Work out the finished part from the listing and answer in its coordinate system (mm). A direction names the side the tool comes from. Coordinates: 2 decimals unless noted, no trailing zeros. Write each loop counter-clockwise with the first axis right and the second up, starting at its lowest first coordinate (ties: lowest second). Pieces come first, ordered by that corner, then holes. Notation, with made-up numbers: (86, 81.25) - (121, 81.25) arc R17 ccw to (121, 102.25) - close; hole circle Ø1 at (-12, -20). An arc over 180 degrees is marked (long way). Use a Markdown table: item, result. Add a question column.
(1) For a pull along Z with two mould halves and no side action, classify faces 4 (the face through (37.236, 8, -89)), 5 (the face through (182.496, 124.457, -88.621)), 6 (the face through (187.325, 89, -83)) as released by +Z, released by -Z, zero draft, split by the parting line, or undercut.
(2) The part is cut by section B-B, the plane y = 84. Give the vertices of the cut face in (x, z) (3 decimals), then the cut area to 3 significant figures.
(3) The part is cut by section A-A, the plane x = 79. Give the vertices of the cut face in (y, z).
(4) A tool of negligible diameter and unlimited length cuts with its end or side. For faces 1 (the face through (185, 52.701, -89)), 2 (the face through (109, 8, -117.196)), 3 (the face through (83, 10.16, -66)), from which of +Z, -Z, +X, -X, +Y, -Y can it reach the whole face along a straight path? Write none if from no direction.
(5) Given pin 1 Ø17.5 at (y, z) = (99.5, -92.5) entering from +X (3 decimals); pin 2 Ø1.9 at (y, z) = (111.76, -88.9) entering from +X; pin 3 Ø12 at (y, z) = (65, -71) entering from -X; pin 4 Ø10 at (x, z) = (150, -111.5) entering from +Y, each flat-ended and moving along its own axis, determine where each tip first touches the part or whether it passes through.
(6) The part is cut by section C-C, the plane z = -139. Give the vertices of the cut face in (x, y), then the cut area to 3 significant figures.
(7) The part is cut by section D-D, the plane x = 23. Give the vertices of the cut face in (y, z).
(8) Find the intervals of material crossed by line 1 (Y direction, x = 185.25, z = -88.9); line 2 (Z direction, x = 39, y = 10); line 3 (Z direction, x = 181.5, y = 111.76), in increasing order. Write a range as from..to.
Autodesk Inventor part; units mm, degrees
ref_plane "Work Plane1" through (177.8, 10.16, -88.9) normal (0, 0, 1) x (1, 0, 0)
ref_plane "YZ Plane" through (0, 0, 0) normal (1, 0, 0) x (0, 1, 0)
ref_plane "XZ Plane" through (0, 0, 0) normal (0, 1, 0) x (-1, 0, 0)
sketch "Sketch1" plane through (0, 0, 0) normal (0, 1, 0) x (-1, 0, 0)
  line L0 (0, 0) -> (-203.2, 0)
  line L1 (-203.2, 0) -> (-203.2, -177.8)
  line L2 (-203.2, -177.8) -> (0, -177.8)
  line L3 (0, -177.8) -> (0, 0)
  dimension "d0" = 203.2
  dimension "d1" = 177.8
extrude "Extrusion1" add sketch "Sketch1" along normal blind 10.16
sketch "Sketch2" plane through (0, 10.16, 0) normal (0, 1, 0) x (1, 0, 0)
  line L0 (203.2, 0) -> (203.2, 177.8)
  line L1 (203.2, 0) -> (177.8, 0)
  line L2 (177.8, 0) -> (177.8, 177.8)
  line L3 (177.8, 177.8) -> (203.2, 177.8)
  line L4 (203.2, 177.8) -> (203.2, 0)
  point P0 (0, 0)
  dimension "d4" = 25.4
extrude "Extrusion2" add sketch "Sketch2" along normal blind 42.5408
sketch "Sketch3" plane through (177.8, 10.16, -177.8) normal (-1, 0, 0) x (0, 0, 1)
  circle A0 centre (88.9, 25.4) radius 10.3886
  line L0 (81.407, 32.5957) -> (96.393, 32.5957)
  line L1 (81.5172, 18.0912) -> (96.2828, 18.0912)
  line L2 (0, 0) -> (177.8, 0)
  line L3 (82.9273, 33.9) -> (94.8727, 33.9)
  line L4 (82.9273, 16.9) -> (94.8727, 16.9)
  point P0 (177.8, -10.16)
  point P1 (88.9, -101.6)
  point P2 (88.8996, -101.6)
  point P3 (100.9466, -114.2832)
  point P4 (102.2534, -114.2832)
  point P5 (114.3004, -101.6)
  point P6 (114.3, -101.6)
  point P7 (159.1068, 0)
  point P8 (88.9, -76.6381)
  point P9 (114.2997, -101.509)
  point P10 (18.6932, 0)
  dimension "d7" = 20.7772
  dimension "d9" = 14.986
  dimension "d45" = 25.4
  dimension "d58" = 8.5
  dimension "d59" = 8.5
extrude "Extrusion3" cut sketch "Sketch3" against normal blind 50.8 contours A0 L1 L0
sketch "Sketch5" plane through (177.8, 10.16, -177.8) normal (-1, 0, 0) x (0, 0, 1)
  line L0 (-12.7, 203.2) -> (190.5, 203.2)
  line L1 (190.5, 203.2) -> (190.5, 0)
  line L2 (-12.7, 0) -> (-12.7, 203.2)
  line L3 (-12.7, 101.6) -> (190.5, 101.6)
  circle A0 centre (88.9, 101.6) radius 1.5635
  circle A1 centre (88.9, 101.6) radius 12.7
  arc A2 (13.581, 0) -> (76.2003, 101.691) centre (-39.021, 102.5166) ccw
  arc A3 (23.8054, 0) -> (88.9, 95.25) centre (-25.9987, 103.9047) ccw
  line L4 (88.9, -246.9942) -> (88.9, 203.2)
  arc A4 (101.5997, 101.691) -> (164.219, 0) centre (216.821, 102.5166) ccw
  arc A5 (88.9, 95.25) -> (153.9946, 0) centre (203.7987, 103.9047) ccw
  line L5 (153.9946, 0) -> (164.219, 0)
  line L6 (13.581, 0) -> (23.8054, 0)
  line L7 (-12.7, 0) -> (190.5, 0)
  line L8 (177.8, 0) -> (0, 0)
  line L9 (177.8, 42.5408) -> (0, 42.5408)
  line L10 (88.9, 42.5408) -> (88.9, 0)
  line L11 (0, 0) -> (177.8, 0)
  line L12 (13.581, 0) -> (-12.7, 0)
  line L13 (164.219, 0) -> (190.5, 0)
  point P0 (177.8, -10.16)
  point P1 (88.9, -101.6)
  point P2 (88.8996, -101.6)
  point P3 (100.9466, -114.2832)
  point P4 (102.2534, -114.2832)
  point P5 (114.3004, -101.6)
  point P6 (114.3, -101.6)
  point P7 (159.1068, 0)
  point P8 (88.9, -21.8971)
  point P9 (114.2997, -101.509)
  point P10 (88.9, 0)
  point P11 (76.2, 101.6)
  point P12 (76.1996, 101.6)
  point P13 (59.3636, 42.5408)
  point P14 (71.5262, 42.5408)
  point P15 (88.2466, 88.9168)
  point P16 (89.5534, 88.9168)
  point P17 (106.2738, 42.5408)
  point P18 (118.4364, 42.5408)
  point P19 (101.6004, 101.6)
  point P20 (101.6, 101.6)
  dimension "d34" = 25.4
  dimension "d31" = 203.2
  dimension "d32" = 203.2
  dimension "d33" = 3.127
  dimension "d35" = 115.2242
  dimension "d36" = 115.2242
  dimension "d37" = 26.281
  dimension "d38" = 6.35
  dimension "d39" = 101.6
  dimension "d40" = 10.2243
extrude "Extrusion4" add sketch "Sketch5" against normal blind 9.525 contours L4 A0 L3 A1 | A1 L3 A0 L4 | L3 A0 L4 A3 A1 | A1 A3 L9 A2 | A3 L4 A1 | A1 A5 L4 A0 L3 | A4 L9 A5 A1 | L4 A5 A1
sketch "Sketch6" plane through (177.8, 10.16, -177.8) normal (-1, 0, 0) x (0, 0, 1)
  arc A0 (13.581, 0) -> (76.2003, 101.691) centre (-39.021, 102.5166) ccw
  arc A1 (101.5997, 101.691) -> (164.219, 0) centre (216.821, 102.5166) ccw
  line L0 (177.8, 0) -> (177.8, 42.5408)
  line L1 (0, 0) -> (177.8, 0)
  line L2 (177.8, 42.5408) -> (0, 42.5408)
  line L3 (0, 0) -> (0, 42.5408)
  arc A2 (13.581, 0) -> (59.3636, 42.5408) centre (-39.021, 102.5166) ccw
  arc A3 (101.6004, 101.6) -> (118.4364, 42.5408) centre (216.821, 102.5166) ccw
  arc A4 (118.4364, 42.5408) -> (164.219, 0) centre (216.821, 102.5166) ccw
  line L4 (0, 42.5408) -> (59.3636, 42.5408)
  line L5 (59.3636, 42.5408) -> (0, 42.5408)
  line L6 (0, 42.5408) -> (0, 0)
  line L7 (177.8, 0) -> (0, 0)
  line L8 (0, 0) -> (13.581, 0)
  line L9 (164.219, 0) -> (177.8, 0)
  line L10 (177.8, 0) -> (177.8, 42.5408)
  line L11 (118.4364, 42.5408) -> (177.8, 42.5408)
  line L12 (118.4364, 42.5408) -> (177.8, 42.5408)
  point P0 (177.8, -10.16)
  point P1 (118.4364, 42.5408)
  point P2 (59.3636, 42.5408)
extrude "Extrusion5" cut sketch "Sketch6" against normal blind 50.8 contours L1 L3 L2 A0 | A1 L2 L0 L1
sketch "Sketch7" plane through (0, 0, 0) normal (0, -1, 0) x (1, 0, 0)
  line L0 (203.2, 0) -> (203.2, -177.8)
  line L1 (0, 0) -> (203.2, 0)
  line L2 (203.2, 0) -> (203.2, -177.8)
  line L3 (203.2, -177.8) -> (0, -177.8)
  line L4 (0, -177.8) -> (0, 0)
extrude "Extrusion6" cut sketch "Sketch7" against normal blind 5.08
sketch "Sketch8" plane through (0, 10.16, -177.8) normal (-1, 0, 0) x (0, 0, 1)
  line L0 (0, -5.08) -> (0, 0)
  line L1 (0, 0) -> (177.8, 0)
  line L2 (177.8, 0) -> (177.8, -5.08)
  line L3 (177.8, -5.08) -> (0, -5.08)
  line L4 (0, -5.08) -> (0, 0)
  point P0 (177.8, -10.16)
extrude "Extrusion7" cut sketch "Sketch8" against normal blind 11.8364
ref_plane "Work Plane1" through (177.8, 10.16, -88.9) normal (0, 0, 1) x (1, 0, 0)
sketch "Sketch9" plane through (0, 5.08, 0) normal (0, -1, 0) x (1, 0, 0)
  line L0 (177.8, -177.8) -> (11.8364, -177.8)
  line L1 (203.2, 0) -> (11.8364, 0)
  line L2 (11.8364, 0) -> (11.8364, -177.8)
  line L3 (11.8364, -177.8) -> (203.2, -177.8)
  line L4 (203.2, -177.8) -> (203.2, 0)
  line L5 (177.8, -177.8) -> (203.2, -177.8)
  line L6 (180.173, -177.8) -> (180.173, -117.1956)
  line L7 (203.2, -59.3636) -> (203.2, -118.4364)
  line L8 (203.2, -117.1956) -> (11.8364, -117.1956)
  line L9 (11.8364, -177.8) -> (11.8364, 0)
  line L10 (155.6362, -177.8) -> (155.6362, -164.211)
  line L11 (177.8, -164.219) -> (203.2, -164.219)
  line L12 (203.2, -164.219) -> (11.8364, -164.219)
  line L13 (102.4836, -164.219) -> (102.4836, -153.9828)
  line L14 (203.2, 0) -> (203.2, -177.8)
  line L15 (203.2, -153.9828) -> (11.8364, -153.9828)
  line L16 (132.8442, -117.1956) -> (132.8442, -110.8456)
  line L17 (203.2, -110.8456) -> (11.8364, -110.8456)
  line L18 (332.5893, -177.8) -> (332.5893, 0)
  line L19 (203.2, -96.2828) -> (203.2, -81.5172)
  line L20 (203.2, -88.9) -> (11.8364, -88.9)
  line L21 (203.2, -60.6044) -> (11.8364, -60.6044)
  line L22 (203.2, -13.581) -> (11.8364, -13.581)
  line L23 (203.2, -23.8172) -> (11.8364, -23.8172)
  line L24 (203.2, -66.9544) -> (11.8364, -66.9544)
  line L25 (177.8, 0) -> (177.8, -177.8)
  line L26 (177.8, 0) -> (177.8, -177.8)
  line L27 (11.8364, -201.1873) -> (37.2364, -201.1873)
  line L28 (37.2364, -177.8) -> (37.2364, 0)
  line L29 (11.8364, 0) -> (177.8, 0)
  point P0 (0, 0)
  point P1 (37.2364, -164.219)
  point P2 (37.2364, -117.1956)
  point P3 (37.2364, -153.9828)
  point P4 (177.8, -153.9828)
  point P5 (177.8, -117.1956)
  point P6 (37.2364, -66.9544)
  point P7 (37.2364, -110.8456)
  point P8 (177.8, -110.8456)
  point P9 (177.8, -66.9544)
  point P10 (37.2364, -23.8172)
  point P11 (37.2364, -60.6044)
  point P12 (177.8, -60.6044)
  point P13 (177.8, -23.8172)
  point P14 (37.2364, 0)
  point P15 (37.2364, -13.581)
  point P16 (177.8, -13.581)
  point P17 (11.8364, -13.581)
  point P18 (11.8364, -164.219)
  point P19 (180.173, -164.219)
  dimension "d51" = 60.6044
  dimension "d52" = 13.589
  dimension "d53" = 10.2362
  dimension "d54" = 6.35
  dimension "d55" = 25.4
extrude "Extrusion8" cut sketch "Sketch9" against normal through all contours L25 L11 L6 L3 | L0 L10 L12 L25 | L0 L28 L12 L10 | L6 L11 L4 L3 | L0 L2 L12 L28 | L15 L28 L8 L25 | L17 L28 L20 L25 | L20 L28 L24 L25 | L21 L28 L23 L25 | L25 L1 L4 L22 | L22 L28 L1 L25 | L22 L2 L1 L28
sketch "Sketch10" plane through (177.8, 111.76, -88.9) normal (-1, 0, 0) x (0, 0, 1)
  arc A0 (7.3828, -83.5088) -> (7.493, -69.0043) centre (0, -76.2) ccw
  circle A1 centre (0, -76.2) radius 10.3886
  line L0 (-16.5091, -76.2) -> (-16.5091, -84.7)
  line L1 (-5.9727, -84.7) -> (5.9727, -84.7)
  line L2 (-16.5091, -76.2) -> (-16.5091, -67.7)
  line L3 (-5.9727, -67.7) -> (10.3883, -67.7)
  line L4 (-7.493, -69.0043) -> (7.493, -69.0043)
  point P0 (88.9, -111.76)
  point P1 (7.493, -69.0043)
  point P2 (5.9727, -67.7)
  point P3 (7.3828, -83.5088)
  dimension "d62" = 8.5
  dimension "d63" = 8.5
extrude "Extrusion9" cut sketch "Sketch10" against normal through all contours A1 L1 L4 A0 | L4 A1 L3
sketch "Sketch11" plane through (203.2, 52.7008, -59.3636) normal (1, 0, 0) x (0, 0, -1)
  line L0 (-65.6844, 19.5873) -> (128.5678, 19.5873)
  line L1 (128.5678, 19.5873) -> (128.5678, -67.3009)
  line L2 (128.5678, -67.3009) -> (-65.6844, -67.3009)
  line L3 (-65.6844, -67.3009) -> (-65.6844, 19.5873)
  point P0 (-59.3636, -52.7008)
extrude "Extrusion10" cut sketch "Sketch11" against normal blind 12.7
properties part number "base plate main"
Model answer:
| question | item | result |
|---|---|---|
| 1 | face 4 | undercut |
| 1 | face 5 | split by the parting line |
| 1 | face 6 | zero draft |
| 2 | outline | (177.8, -105.222) - (187.325, -105.222) - (187.325, -92.566) - (177.8, -92.566) - close; (177.8, -85.234) - (187.325, -85.234) - (187.325, -72.578) - (177.8, -72.578) - close |
| 2 | area | 241 mm^2 |
| 3 | outline | (5.08, -164.22) - (10.16, -164.22) - (10.16, -153.98) - (5.08, -153.98) - close; (5.08, -117.2) - (10.16, -117.2) - (10.16, -110.85) - (5.08, -110.85) - close; (5.08, -66.95) - (10.16, -66.95) - (10.16, -60.6) - (5.08, -60.6) - close; (5.08, -23.82) - (10.16, -23.82) - (10.16, -13.58) - (5.08, -13.58) - close |
| 4 | face 1 | +X |
| 4 | face 2 | +Y, -Y |
| 4 | face 3 | +Z, -Z, -X, +Y |
| 5 | pin 1 | x = 187.325 |
| 5 | pin 2 | through |
| 5 | pin 3 | x = 177.8 |
| 5 | pin 4 | y = 10.16 |
| 6 | outline | (11.84, 5.08) - (37.24, 5.08) - (37.24, 10.16) - (11.84, 10.16) - close; (177.8, 5.08) - (190.5, 5.08) - (190.5, 27.7) - (177.8, 27.7) - close |
| 6 | area | 416 mm^2 |
| 7 | outline | (5.08, -164.22) - (10.16, -164.22) - (10.16, -13.58) - (5.08, -13.58) - close |
| 8 | line 1 | 5.08..27.06, 44.06..52.7, 99.06..110.2, 113.32..124.46 |
| 8 | line 2 | -164.22..-153.98, -117.2..-110.85, -66.95..-60.6, -23.82..-13.58 |
| 8 | line 3 | -101.6..-90.46, -87.34..-76.2 |
